from build123d import *

# Parameters (mm, degrees)
F1_W     = 240
F1_H     = 240
F1_W_2   = 6
F1_H_2   = 6
F1_W_3   = 208
F1_H_3   = 208
F2_DEPTH = 3
F3_DEPTH = 25
F8_W     = 6
F8_H     = 6
F8_W_2   = 16
F8_H_2   = 208
F9_DEPTH = 3.001


with BuildPart() as f2:
    # F1 (on Front) → F2 (new body)
    with BuildSketch(Plane.XZ):
        with Locations((120, 120)):
            Rectangle(F1_W, F1_H)
        with Locations((6, 234)):
            Rectangle(F1_W_2, F1_H_2, mode=Mode.SUBTRACT)
        with Locations((120, 120)):
            Rectangle(F1_W_3, F1_H_3, mode=Mode.SUBTRACT)
        with Locations((6, 234)):
            Rectangle(F1_W_2, F1_H_2)
    extrude(amount=F2_DEPTH)

    # F1 (on Front) → F3 (cut)
    with BuildSketch(Plane.XZ):
        with Locations((6, 234)):
            Rectangle(F1_W_2, F1_H_2)
    extrude(amount=F3_DEPTH, mode=Mode.SUBTRACT)

    # F5: F2 across plane


with BuildPart() as f2_1:
    add(f2.part)
    add(f2.part.mirror(Plane(origin=(120, -1.5, 120), x_dir=(0, -1, 0), z_dir=(-1, 0, 0))), mode=Mode.INTERSECT)

    # F7: F2 across plane


with BuildPart() as f2_2:
    add(f2_1.part)
    add(f2_1.part.mirror(Plane(origin=(120, -1.5, 120), x_dir=(1, 0, 0), z_dir=(0, 0, 1))), mode=Mode.INTERSECT)

    # F8 (on face) → F9 (cut, through all)
    with BuildSketch(Plane.XZ.offset(3)):
        Polygon((240, 240), (0, 240), (0, 224), (16, 224), (224, 224), (240, 224), align=None)
        with Locations((6, 234)):
            Rectangle(F8_W, F8_H, mode=Mode.SUBTRACT)
        with Locations((234, 234)):
            Rectangle(F8_W, F8_H, mode=Mode.SUBTRACT)
        with Locations((232, 120)):
            Rectangle(F8_W_2, F8_H_2)
    extrude(amount=-F9_DEPTH, mode=Mode.SUBTRACT)


solid = f2_2.part
CAD build for the part. Positions are in the model's coordinates, mm. Round coordinates to 2 decimals unless told otherwise and drop trailing zeros. Order: outer loops, then holes, each group sorted by start corner. A loop starts at its lowest first (then second) coordinate and runs counter-clockwise, first axis right, second up. Notation, with made-up numbers: M 20,68 L 33,68 A13 ccw 33,90 Z; hole C 3.5,78.5 d9. An arc over 180 degrees is marked long. Use one line per item in the form item = value.
Q1. Probe L1, parallel to X at y = -0.8, z = 36. List the from-to ranges inside material, lowest first.
Recorded:
L1 = 0 to 16
Q2. Saw through at B-B on z = 193.5. Give the cut face in (x, y).
Recorded:
outline = M 0,-3 L 16,-3 L 16,0 L 0,0 Z
Q3. Flat gauge pins, fed straight in: P1, Ø1.5, axis at x = 234.5, y = -2, coming from the -Z side; P2, Ø1.5, axis at y = -2, z = 98.5, coming from the +X side; P3, Ø0.9, axis at x = 234, y = -1, coming from the +Z side. Where does each tip first touch, or does it go through?
Recorded:
P1 = 0
P2 = 16
P3 = 16
Q4. Saw through at A-A on y = -2.3. Give the cut face in (x, z), then the cut area to 3 significant figures.
Recorded:
outline = M 0,0 L 240,0 L 240,16 L 16,16 L 16,224 L 0,224 Z; hole M 3,3 L 9,3 L 9,9 L 3,9 Z; hole M 231,3 L 237,3 L 237,9 L 231,9 Z
area = 7,100 mm^2
Q5. Saw through at C-C on x = 75.5. Give the cut face in (y, z), then the cut area to 3 significant figures.
Recorded:
outline = M -3,0 L 0,0 L 0,16 L -3,16 Z
area = 48.0 mm^2
